Input: part model. Units: mm. Frame: model coordinates. Face numbers are marked on the shaded views. Give positions to 0.01 mm unless a question says otherwise; leave off trailing zeros. Loops run counter-clockwise (first coordinate to the right, second up) from the corner with the lowest first, then second, coordinate; pieces in that order, holes last. Notation, with made-up numbers: M 16,62 L 75,62 A18 ccw 75,72 Z; hole C 12,-10.5 d5. An arc over 180 degrees is marked long. Return JSON: item names as keys, results as strings. Group by question number.
```python
from build123d import *

# Parameters (mm, degrees)
F0_R     = 38.5
F0_R_2   = 36
F1_DEPTH = 5
F2_R     = 38.5
F2_R_2   = 36
F2_R_3   = 34
F3_DEPTH = 4
F4_R     = 38.5
F4_R_2   = 37.5
F5_DEPTH = 5
F6_R     = 38.5
F6_R_2   = 34
F7_DEPTH = 3


with BuildPart() as f1:
    # F0 (on Top) → F1 (new body)
    with BuildSketch(Plane.XY):
        Circle(F0_R)
        Circle(F0_R_2, mode=Mode.SUBTRACT)
    extrude(amount=F1_DEPTH)

    # F2 (on face) → F3 (join)
    with BuildSketch(Plane.XY.offset(5)):
        Circle(F2_R)
        Circle(F2_R_2, mode=Mode.SUBTRACT)
        Circle(F2_R_2)
        Circle(F2_R_3, mode=Mode.SUBTRACT)
    extrude(amount=F3_DEPTH)

    # F4 (on face) → F5 (join)
    with BuildSketch(Plane.XY.offset(9)):
        Circle(F4_R)
        Circle(F4_R_2, mode=Mode.SUBTRACT)
    extrude(amount=F5_DEPTH)

    # F6 (on face) → F7 (join)
    with BuildSketch(Plane.XY.offset(14)):
        Circle(F6_R)
        Circle(F6_R_2, mode=Mode.SUBTRACT)
    extrude(amount=F7_DEPTH)


solid = f1.part
```
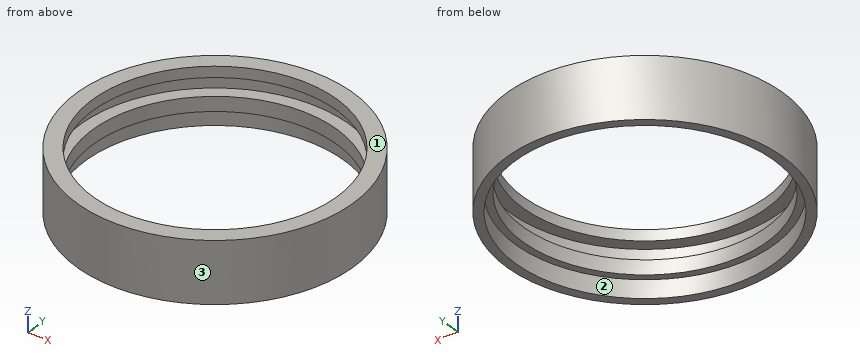
Item 1: Section D-D, the plane z = 2. Return loops of the section in (x, y), then the cut area to 3 significant figures.
Item 2: Pull-direction query (X, two-part tool) for the marked faces 1, 2 and 3; classes: pulls with the +X half, pulls with the -X half, needs draft (parallel to the pull), parting line crosses it, or undercut.
Item 3: Section C-C, the plane z = 13. Return loops of the section in (x, y), then the cut area to 3 significant figures.
Item 4: Section A-A, the plane y = 0. Return loops of the section in (x, z), then the cut area to 3 significant figures.
Item 5: First-contact query: pin 1 Ø3 at (y, z) = (-27.5, 6) entering from -X; pin 2 Ø1 at (x, z) = (18.5, 14) entering from +Y; pin 3 Ø2 at (x, z) = (24.5, 2) entering from -Y. Flat tips, straight axial feed; report the tip coordinate or a pass-through.
Item 6: Material intervals for line 1 (Y direction, x = 0, z = 3.5); line 2 (Y direction, x = 0, z = 6.4); line 3 (X direction, y = 1, z = 16), sorted ascending. Write a range as from..to.
Answer below:
{
 "1": {"outline": "C 0,0 d77; hole C 0,0 d72", "area": "585 mm^2"},
 "2": {"face 1": "needs draft", "face 2": "undercut", "face 3": "parting line crosses it"},
 "3": {"outline": "C 0,0 d77; hole C 0,0 d75", "area": "239 mm^2"},
 "4": {"outline": "M -38.5,0 L -36,0 L -36,5 L -34,5 L -34,9 L -37.5,9 L -37.5,14 L -34,14 L -34,17 L -38.5,17 Z; M 34,5 L 36,5 L 36,0 L 38.5,0 L 38.5,17 L 34,17 L 34,14 L 37.5,14 L 37.5,9 L 34,9 Z", "area": "98.0 mm^2"},
 "5": {"pin 1": "x = -28.39", "pin 2": "y = 34.03", "pin 3": "y = -30.5"},
 "6": {"line 1": "-38.5..-36, 36..38.5", "line 2": "-38.5..-34, 34..38.5", "line 3": "-38.49..-33.99, 33.99..38.49"}
}
